```python
from build123d import *

# Parameters (mm, degrees)
CHAMFER001_SIZE    = 3
SKETCH013_R        = 0.4
PAD008_DEPTH       = 12.5
POLARPATTERN_COUNT = 11
POLARPATTERN_ANGLE = 330


with BuildPart() as part:
    # Sketch012 → Revolution (revolve)
    with BuildSketch(Plane.XZ):
        with BuildLine():
            Line((0, 55), (0, 0))
            Line((0, 0), (11, 0))
            Line((11, 0), (11, 45))
            add(Edge.make_bspline(
                [(0, 55), (0, 50.541328), (11, 53.4418), (11, 45)],
                knots=[0, 0, 0, 0, 1, 1, 1, 1], degree=3))
        make_face()
    revolve(axis=Axis((0, 0, 0), (0, 0, 1)))

    # Chamfer001
    chamfer001_edges = [part.edges().sort_by_distance(p)[0] for p in [
        (-11, 0, 0),
    ]]
    chamfer(chamfer001_edges, length=CHAMFER001_SIZE)

    # Sketch013 (on Face1 of Revolution) → Pad008 (new body)
    with BuildSketch(Plane(origin=(0, 0, 0), x_dir=(1, 0, 0), z_dir=(0, 0, -1))):
        with Locations((6, 0)):
            Circle(SKETCH013_R)
    pad008 = extrude(amount=PAD008_DEPTH)

    # PolarPattern: Pad008 ×11 about axis
    polarpattern_axis = Axis((0, 0, 0), (0, 0, -1))
    for i in range(1, POLARPATTERN_COUNT):
        add(pad008.rotate(polarpattern_axis, i * POLARPATTERN_ANGLE / (POLARPATTERN_COUNT - 1)))


with BuildPart() as part_1:
    # Body002 placement: moved
    add(part.part.moved(Location((4, 19, 0))))


solid = part_1.part
```
Verification items for the finished model (mm, model axes). Round coordinates to 2 decimals unless told otherwise and drop trailing zeros. Order: outer loops, then holes, each group sorted by start corner. A loop starts at its lowest first (then second) coordinate and runs counter-clockwise, first axis right, second up.
1) Material ranges on line 1 (Y direction, x = 9, z = -6); line 2 (Z direction, x = 0.75, y = 15); line 3 (Z direction, x = 11.5, y = 19), recorded low to high.
Geometry says:
line 1: y = 15.33 to 16.13, 21.65 to 22.35
line 2: z = 0 to 51.6
line 3: z = 0 to 50.71
2) Depth check by flat-ended pin: pin 1 (8 mm diameter, centred on x = 7, y = 24, fed in from +Z); pin 2 (1.5 mm diameter, centred on x = -2, y = 27, fed in from +Z); pin 3 (5 mm diameter, centred on y = 22.5, z = -1, fed in from -X). Enter the tip coordinate at first touch or a pass-through.
Geometry says:
pin 1: stops at z = 52.69
pin 2: stops at z = 49.53
pin 3: stops at x = -4.97
3) Cross-section at A-A, the plane z = 41. Record the cut outline in (x, y), plus the area to 3 significant figures.
Geometry says:
outline: circle Ø22 at (4, 19)
area: 380 mm2
